from build123d import *

# Parameters (mm, degrees)
BASE_EXTRUDE_DEPTH  = 8.8
SKETCH3_R           = 7
BOSS_EXTRUDE1_DEPTH = 40
CHAMFER1_SIZE       = 2


with BuildPart() as part:
    # Sketch1 → Base-Extrude (new body)
    with BuildSketch(Plane.XY):
        Polygon((-6.062177826, 10.5), (6.062177826, 10.5), (12.124355653, 0), (6.062177826, -10.5), (-6.062177826, -10.5), (-12.124355653, 0), align=None)
    extrude(amount=BASE_EXTRUDE_DEPTH)

    # Sketch3 → Boss-Extrude1 (add)
    with BuildSketch(Plane(origin=(0, 0, 0), x_dir=(-1, 0, 0), z_dir=(0, 0, -1))):
        with Locations(Location((0, 0, 0), (0, 0, 180))):
            Circle(SKETCH3_R)
    extrude(amount=BOSS_EXTRUDE1_DEPTH)

    # Chamfer1
    chamfer1_edges = [part.edges().sort_by_distance(p)[0] for p in [
        (-7, 0, -40),
    ]]
    chamfer(chamfer1_edges, length=CHAMFER1_SIZE)


solid = part.part
The listing builds one solid part. Answer for the finished solid, in the listing's coordinates (mm). A direction names the side the tool comes from. Coordinates: 2 decimals unless noted, no trailing zeros. Write each loop counter-clockwise with the first axis right and the second up, starting at its lowest first coordinate (ties: lowest second). Pieces come first, ordered by that corner, then holes. Notation, with made-up numbers: M 6.25,81.25 L 22.25,81.25 A35 ccw 22.25,120.25 Z; hole C 40.25,-13 d2. An arc over 180 degrees is marked long. Put each result on its own line as item: value. Start each with the question number.
1. A cutting plane is placed at D-D on x = -8.75. Write down the section's boundary in (y, z).
2. A cutting plane is placed at B-B on z = -36. Write down the section's boundary in (x, y), then the cut area to 3 significant figures.
3. A cutting plane is placed at A-A on x = 0. Write down the section's boundary in (y, z), then the cut area to 3 significant figures.
4. Which of the six approach directions +Z, -Z, +X, -X, +Y, -Y give full straight-line access (tool end or side, diameter ignored) to faces 1 (the flat face through (0, 0, 8.8)), 2 (the cylindrical face through (6.466, 2.681, -18.734))?
5. Consider line 1 (Z direction, x = -6.25, y = -4); line 2 (X direction, y = 0.25, z = -1.5); line 3 (Z direction, x = -0.75, y = 5). Determine where each line is inside the solid, lowest interval first. Write a range as from..to.
6. A cutting plane is placed at C-C on z = 1. Write down the section's boundary in (x, y), then the cut area to 3 significant figures.
7. Flat-ended cylindrical pins translate along their axes: P1, Ø3, axis at y = 0, z = -6.5, coming from the -X side; P2, Ø1, axis at y = 3, z = -25, coming from the -X side; P3, Ø2, axis at x = 0.5, z = -22.5, coming from the +Y side. Find the tip coordinate at first contact, or state that the pin passes through.
Resolved:
1. outline: M -5.84,0 L 5.84,0 L 5.84,8.8 L -5.84,8.8 Z
2. outline: C 0,0 d14
2. area: 154 mm2
3. outline: M -10.5,0 L -7,0 L -7,-38 L -5,-40 L 5,-40 L 7,-38 L 7,0 L 10.5,0 L 10.5,8.8 L -10.5,8.8 Z
3. area: 741 mm2
4. face 1: +Z, +X, -X, +Y, -Y
4. face 2: -Z
5. line 1: z = 0..8.8
5. line 2: x = -7..7
5. line 3: z = -39.94..8.8
6. outline: M -12.12,0 L -6.06,-10.5 L 6.06,-10.5 L 12.12,0 L 6.06,10.5 L -6.06,10.5 Z
6. area: 382 mm2
7. P1: stops at x = -7
7. P2: stops at x = -6.54
7. P3: stops at y = 7
